```python
from build123d import *

# Parameters (mm, degrees)
SKETCH1_R           = 3.5
BOSS_EXTRUDE1_DEPTH = 5
SKETCH2_R           = 2.5
BOSS_EXTRUDE2_DEPTH = 50
BOSS_EXTRUDE3_START = 5
SKETCH3_R           = 3.5
BOSS_EXTRUDE3_DEPTH = 5
FILLET1_R           = 0.5


with BuildPart() as part:
    # Sketch1 → Boss-Extrude1 (new body)
    with BuildSketch(Plane.XY):
        Circle(SKETCH1_R)
    extrude(amount=BOSS_EXTRUDE1_DEPTH)

    # Sketch2 → Boss-Extrude2 (add)
    with BuildSketch(Plane(origin=(0, 0, 0), x_dir=(-1, 0, 0), z_dir=(0, 0, -1))):
        with Locations(Location((0, 0, 0), (0, 0, 180))):
            Circle(SKETCH2_R)
    extrude(amount=BOSS_EXTRUDE2_DEPTH)

    # Sketch3 → Boss-Extrude3 (add)
    with BuildSketch(Plane(origin=(0, 0, -50), x_dir=(-1, 0, 0), z_dir=(0, 0, -1)).offset(BOSS_EXTRUDE3_START)):
        with Locations(Location((0, 0, 0), (0, 0, 180))):
            Circle(SKETCH3_R)
    extrude(amount=-BOSS_EXTRUDE3_DEPTH)

    # Fillet1
    fillet1_edges = [part.edges().sort_by_distance(p)[0] for p in [
        (-3.5, 0, 0),
        (-3.5, 0, 5),
        (-3.5, 0, -50),
        (-3.5, 0, -55),
    ]]
    fillet(fillet1_edges, radius=FILLET1_R)


solid = part.part
```
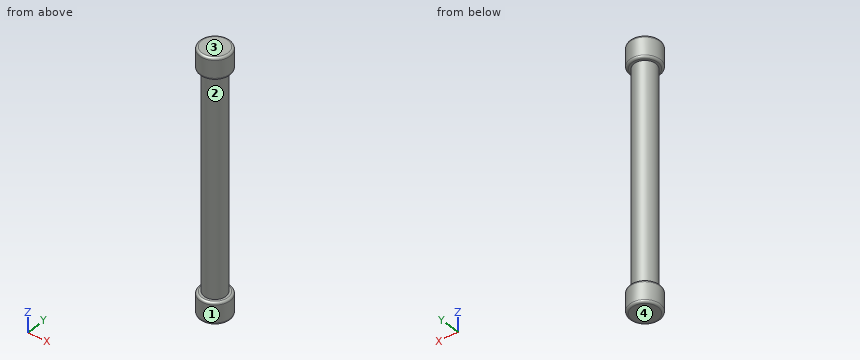
CAD build for the part. Positions are in the model's coordinates, mm. Face numbers are marked on the shaded views. Coordinates: 2 decimals unless noted, no trailing zeros. Write each loop counter-clockwise with the first axis right and the second up, starting at its lowest first coordinate (ties: lowest second). Pieces come first, ordered by that corner, then holes. Notation, with made-up numbers: (85.5, 9) -> (137.5, 9) arc R26 cw to (137.5, 38) -> close; hole circle Ø2 at (31, 51.5). An arc over 180 degrees is marked (long way). Return JSON: item names as keys, results as strings. Group by question number.
Q1. Drill centre lines: line 1 (Z direction, x = 1.75, y = -2.5); line 2 (Z direction, x = 1.75, y = 2.75); line 3 (Y direction, x = -0.25, z = -39.5). Where is each one in solid material? Low to high.
Q2. Pull direction Z, two halves, no side cores. Call the marked faces 1, 2, 3 and 4: released by +Z, released by -Z, zero draft, split by the parting line, or undercut.
Q3. Flat gauge pins, fed straight in: pin 1 (1.5 mm diameter, centred on y = -3, z = -22.5, fed in from -X); pin 2 (1 mm diameter, centred on x = -1, z = -13.5, fed in from -Y); pin 3 (1.5 mm diameter, centred on x = 2.5, z = -29, fed in from +Y). Where does each tip first touch, or does it go through?
Q4. Cut at C-C, the plane z = -51. Give the cut face in (x, y), then the cut area to 3 significant figures.
Q5. Cut at D-D, the plane z = -29. Give the cut face in (x, y).
Q6. Cut at A-A, the plane y = 0. Give the cut face in (x, z), then the cut area to 3 significant figures.
Returned:
{
 "1": {"line 1": "z = -55 to -50, 0 to 5", "line 2": "z = -54.93 to -50.07, 0.07 to 4.93", "line 3": "y = -2.49 to 2.49"},
 "2": {"face 1": "zero draft", "face 2": "undercut", "face 3": "released by +Z", "face 4": "released by -Z"},
 "3": {"pin 1": "stops at x = -1.09", "pin 2": "stops at y = -2.45", "pin 3": "stops at y = 1.79"},
 "4": {"outline": "circle Ø7 at (0, 0)", "area": "38.5 mm2"},
 "5": {"outline": "circle Ø5 at (0, 0)"},
 "6": {"outline": "(-3.5, -54.5) arc R0.5 ccw to (-3, -55) -> (3, -55) arc R0.5 ccw to (3.5, -54.5) -> (3.5, -50.5) arc R0.5 ccw to (3, -50) -> (2.5, -50) -> (2.5, 0) -> (3, 0) arc R0.5 ccw to (3.5, 0.5) -> (3.5, 4.5) arc R0.5 ccw to (3, 5) -> (-3, 5) arc R0.5 ccw to (-3.5, 4.5) -> (-3.5, 0.5) arc R0.5 ccw to (-3, 0) -> (-2.5, 0) -> (-2.5, -50) -> (-3, -50) arc R0.5 ccw to (-3.5, -50.5) -> close", "area": "320 mm2"}
}
